from build123d import *

# Parameters (mm, degrees)
F0_R     = 4.953
F0_R_2   = 21.4376
F1_DEPTH = 12.7


with BuildPart() as f1:
    # F0 (on Front) → F1 (new body, symmetric)
    with BuildSketch(Plane.XZ):
        with BuildLine():
            Line((59.3833293236, -10.6172418004), (34.4828311796, 49.4978785287))
            ThreePointArc((34.4828311796, 49.4978785287), (0, 60.325), (-34.4828311796, 49.4978785287))
            Line((-34.4828311796, 49.4978785287), (-59.3833293236, -10.6172418004))
            ThreePointArc((-59.3833293236, -10.6172418004), (0, -60.325), (59.3833293236, -10.6172418004))
        make_face()
        with Locations((0, -46.101)):
            Circle(F0_R, mode=Mode.SUBTRACT)
        Circle(F0_R_2, mode=Mode.SUBTRACT)
        with Locations((0, 46.101)):
            Circle(F0_R, mode=Mode.SUBTRACT)
    extrude(amount=F1_DEPTH, both=True)


solid = f1.part
Could you check a few things on this model? Use its own coordinates, in mm. Give positions to 0.01 mm unless a question says otherwise; leave off trailing zeros. Order: outer loops, then holes, each group sorted by start corner. A loop starts at its lowest first (then second) coordinate and runs counter-clockwise, first axis right, second up.
Item 1: If we section it at D-D, the plane y = -6.5: Write out the boundary of the cut face in (x, z) (3 decimals).
Item 2: I'm going to push flat-ended pins straight in: pin 1 (4 mm diameter, centred on x = -13.5, y = 0.5, fed in from +Z); pin 2 (5 mm diameter, centred on x = -17, y = -9.5, fed in from -Z); pin 3 (4 mm diameter, centred on y = 5.5, z = -37.5, fed in from +X). Where does each tip first touch, or does it pass through?
Item 3: If we section it at A-A, the plane z = -5: Write out the boundary of the cut face in (x, y).
Item 4: If we mould it in two halves opening along Z, with no side actions, what happens to faces 1 (the face through (-1, 12.7, -26)), 2 (the face through (-1.177, -0.178, -60.314)), 3 (the face through (-46.76, -0.18, 19.86)), 4 (the face through (-1.074, 0.178, -50.936))? For each: pulls with the +Z half, pulls with the -Z half, needs draft (parallel to the pull), parting line crosses it, or undercut.
Item 5: If we section it at C-C, the plane x = -17.5: Write out the boundary of the cut face in (y, z).
Item 6: I need wall thicknesses on line 1 (Z direction, x = 0, y = 4.5) (3 decimals); line 2 (Z direction, x = -0.5, y = -2.5); line 3 (X direction, y = -4.75, z = 18.5). Which ranges of each line are inside material? Lowest first, please.
Item 7: If we section it at B-B, the plane x = 0: Write out the boundary of the cut face in (y, z) (3 decimals), plus the area to 3 significant figures.
Values:
1. outline: (-59.383, -10.617) arc R60.325 ccw to (59.383, -10.617) - (34.483, 49.498) arc R60.325 ccw to (-34.483, 49.498) - close; hole circle Ø42.875 at (0, 0); hole circle Ø9.906 at (0, -46.101); hole circle Ø9.906 at (0, 46.101)
2. pin 1: stops at z = 59.22
2. pin 2: stops at z = -58.56
2. pin 3: stops at x = 48.77
3. outline: (-57.06, -12.7) - (-20.85, -12.7) - (-20.85, 12.7) - (-57.06, 12.7) - close; (20.85, -12.7) - (57.06, -12.7) - (57.06, 12.7) - (20.85, 12.7) - close
4. face 1: needs draft
4. face 2: pulls with the -Z half
4. face 3: pulls with the +Z half
4. face 4: undercut
5. outline: (-12.7, -57.73) - (12.7, -57.73) - (12.7, -12.38) - (-12.7, -12.38) - close; (-12.7, 12.38) - (12.7, 12.38) - (12.7, 57.73) - (-12.7, 57.73) - close
6. line 1: z = -60.325 to -51.054, -41.148 to -21.438, 21.438 to 41.148, 51.054 to 60.325
6. line 2: z = -60.32 to -51.03, -41.17 to -21.43, 21.43 to 41.17, 51.03 to 60.32
6. line 3: x = -47.32 to -10.83, 10.83 to 47.32
7. outline: (-12.7, -60.325) - (12.7, -60.325) - (12.7, -51.054) - (-12.7, -51.054) - close; (-12.7, -41.148) - (12.7, -41.148) - (12.7, -21.438) - (-12.7, -21.438) - close; (-12.7, 21.438) - (12.7, 21.438) - (12.7, 41.148) - (-12.7, 41.148) - close; (-12.7, 51.054) - (12.7, 51.054) - (12.7, 60.325) - (-12.7, 60.325) - close
7. area: 1,470 mm2
